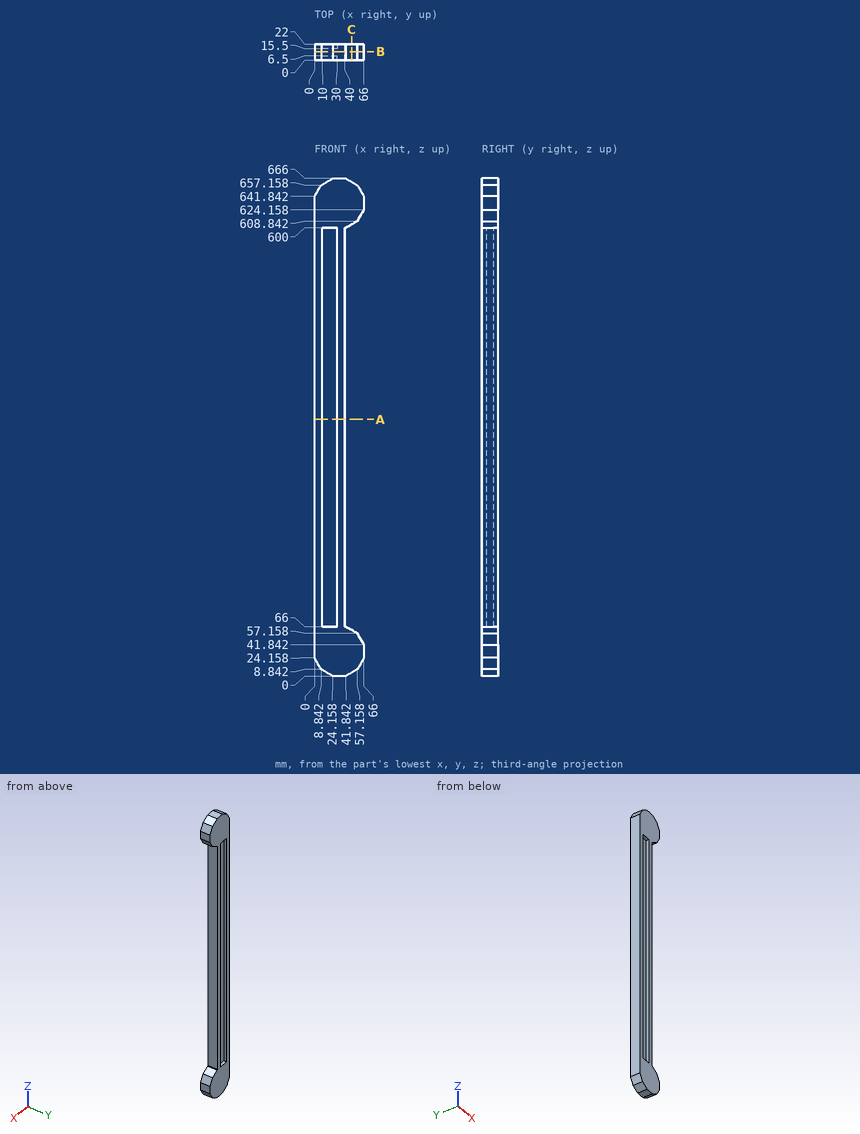
Check sheet for the drawn part. Datum: minimum x, y, z corner. Units: mm. Give positions to 0.01 mm unless a question says otherwise; leave off trailing zeros. Loops run counter-clockwise (first coordinate to the right, second up) from the corner with the lowest first, then second, coordinate; pieces in that order, holes last. Notation, with made-up numbers: M -38.75,24.25 L -34.75,24.25 A14 cw -34.75,29.25 Z; hole C 16,-19.75 d2. An arc over 180 degrees is marked long. Return JSON: item names as keys, results as strings.
1) Section check A-A, the plane z = 343.5. Enter the section's corners in (x, y), and give its area (3 significant figures).
Findings:
{"outline": "M 0,0 L 10,0 L 10,6.5 L 30,6.5 L 30,0 L 40,0 L 40,22 L 30,22 L 30,15.5 L 10,15.5 L 10,22 L 0,22 Z", "area": "620 mm2"}
2) Gauge pin test, flat ends, axial feed: P1, Ø2, axis at y = 18.5, z = 452.5, coming from the +X side; P2, Ø6, axis at x = 58.5, y = 2.5, coming from the -Z side (1 decimal); P3, Ø10, axis at x = 23, z = 404, coming from the +Y side. Record the tip position at first contact, or that the pin passes through.
Findings:
{"P1": "stops at x = 40", "P2": "stops at z = 7.9", "P3": "stops at y = 15.5"}
3) Section check C-C, the plane x = 49.5. Enter the section's corners in (y, z).
Findings:
{"outline": "M 0,4.42 L 22,4.42 L 22,61.58 L 0,61.58 Z; M 0,604.42 L 22,604.42 L 22,661.58 L 0,661.58 Z"}
4) Section check B-B, the plane y = 11.75. Enter the section's corners in (x, z), and give its area (3 significant figures).
Findings:
{"outline": "M 0,24.16 L 8.84,8.84 L 24.16,0 L 41.84,0 L 57.16,8.84 L 66,24.16 L 66,41.84 L 57.16,57.16 L 41.84,66 L 40,66 L 40,600 L 41.84,600 L 57.16,608.84 L 66,624.16 L 66,641.84 L 57.16,657.16 L 41.84,666 L 24.16,666 L 8.84,657.16 L 0,641.84 Z", "area": "28,800 mm2"}
5) Material ranges on L1, parallel to X at y = 16.5, z = 380.5; L2, parallel to Z at x = 41.5, y = 15; L3, parallel to X at y = 7.75, z = 244.5, recorded low to high. Write a range as [from, to].
Findings:
{"L1": "x = [0, 10], [30, 40]", "L2": "z = [0, 66], [600, 666]", "L3": "x = [0, 40]"}
